from build123d import *

# Parameters (mm, degrees)
SKETCH1_R           = 20.6375
BOSS_EXTRUDE1_DEPTH = 3.175
BOSS_EXTRUDE2_START = -3.175
SKETCH2_R           = 14.2875
BOSS_EXTRUDE2_DEPTH = 47.498
SKETCH3_R           = 1.4732
CUT_EXTRUDE1_DEPTH  = 54.069210862
SKETCH4_R           = 13.6144
CUT_EXTRUDE2_DEPTH  = 46.8122
FILLET1_R           = 1.5875


with BuildPart() as part:
    # Sketch1 → Boss-Extrude1 (new body)
    with BuildSketch(Plane(origin=(0, 0, 0), x_dir=(1, 0, 0), z_dir=(0, 1, 0))):
        with Locations(Location((0, 0, 0), (0, 0, 270))):
            Circle(SKETCH1_R)
    extrude(amount=BOSS_EXTRUDE1_DEPTH)

    # Sketch2 → Boss-Extrude2 (add)
    with BuildSketch(Plane(origin=(0, 3.175, 0), x_dir=(1, 0, 0), z_dir=(0, 1, 0)).offset(BOSS_EXTRUDE2_START)):
        with Locations(Location((0, 0, 0), (0, 0, 90))):
            Circle(SKETCH2_R)
    extrude(amount=BOSS_EXTRUDE2_DEPTH)

    # Sketch3 → Cut-Extrude1 (cut, through all)
    with BuildSketch(Plane(origin=(0, 3.175, 0), x_dir=(1, 0, 0), z_dir=(0, 1, 0))):
        with Locations(Location((0, 17.0688, 0), (0, 0, 270))):
            Circle(SKETCH3_R)
        with Locations(Location((14.782014412, -8.5344, 0), (0, 0, 270))):
            Circle(SKETCH3_R)
        with Locations(Location((-14.782014412, -8.5344, 0), (0, 0, 270))):
            Circle(SKETCH3_R)
    extrude(amount=-CUT_EXTRUDE1_DEPTH, mode=Mode.SUBTRACT)

    # Sketch4 → Cut-Extrude2 (cut)
    with BuildSketch(Plane.XZ):
        with Locations(Location((0, 0, 0), (0, 0, 270))):
            Circle(SKETCH4_R)
    extrude(amount=-CUT_EXTRUDE2_DEPTH, mode=Mode.SUBTRACT)

    # Fillet1
    fillet1_edges = [part.edges().sort_by_distance(p)[0] for p in [
        (0, 47.498, 14.2875),
    ]]
    fillet(fillet1_edges, radius=FILLET1_R)


solid = part.part
Geometry: final body of the model. Coordinates: model frame, mm. A direction names the side the tool comes from. Coordinates: 2 decimals unless noted, no trailing zeros. Order: outer loops, then holes, each group sorted by start corner. A loop starts at its lowest first (then second) coordinate and runs counter-clockwise, first axis right, second up.
(1) First-contact query: pin 1 (5 mm diameter, centred on y = 38, z = -6, fed in from -X); pin 2 (4 mm diameter, centred on x = 0, z = 6, fed in from -Y); pin 3 (6 mm diameter, centred on y = 37.5, z = -8.5, fed in from +X). Flat tips, straight axial feed; report the tip coordinate or a pass-through.
(2) Section query B-B (z = 0). Return the cut outline in (x, y) (1 decimal).
(3) Access query for faces 4 (the face through (20.46, 1.57, -2.69)), 5 (the face through (0, 46.812, 0)). Directions: +Z, -Z, +X, -X, +Y, -Y. A direction counts if a zero-diameter tool reaches every point of the face in a straight line with its end or side. Return the directions, or none.
(4) Material intervals for probe 1 along X at (y, z) = (41, 0); probe 2 along Z at (x, y) = (-5, 42.5); probe 3 along Y at (x, z) = (12, 0), sorted ascending.
(5) Draft query along X for faces 1 (the face through (13.5, 23.08, 1.77)), 2 (the face through (-4, 3.175, -14)), 3 (the face through (-0.628, 24.244, 14.274)). Return one class per face: pulls with the +X half, pulls with the -X half, needs draft (parallel to the pull), parting line crosses it, or undercut.
(6) Section query C-C (y = 31.5). Return the cut outline in (x, z) (1 decimal).
(7) Section query A-A (x = 0). Return the cut outline in (y, z) (1 decimal), plus the area to 3 significant figures.
Solution:
1. pin 1: stops at x = -13.85
1. pin 2: stops at y = 46.81
1. pin 3: stops at x = 13.19
2. outline: (-20.6, 0) - (-13.6, 0) - (-13.6, 46.8) - (13.6, 46.8) - (13.6, 0) - (20.6, 0) - (20.6, 3.2) - (14.3, 3.2) - (14.3, 45.9) arc R1.6 ccw to (12.7, 47.5) - (-12.7, 47.5) arc R1.6 ccw to (-14.3, 45.9) - (-14.3, 3.2) - (-20.6, 3.2) - close
3. face 4: +Y, -Y
3. face 5: -Y
4. probe 1: x = -14.29 to -13.61, 13.61 to 14.29
4. probe 2: z = -13.38 to -12.66, 12.66 to 13.38
4. probe 3: y = 46.81 to 47.5
5. face 1: undercut
5. face 2: needs draft
5. face 3: parting line crosses it
6. outline: circle Ø28.6 at (0, 0); hole circle Ø27.2 at (0, 0)
7. outline: (0, -20.6) - (3.2, -20.6) - (3.2, -18.5) - (0, -18.5) - close; (0, -15.6) - (3.2, -15.6) - (3.2, -14.3) - (45.9, -14.3) arc R1.6 ccw to (47.5, -12.7) - (47.5, 12.7) arc R1.6 ccw to (45.9, 14.3) - (3.2, 14.3) - (3.2, 20.6) - (0, 20.6) - (0, 13.6) - (46.8, 13.6) - (46.8, -13.6) - (0, -13.6) - close
7. area: 113 mm2
